Input: part model. Units: mm. Frame: model coordinates. A direction names the side the tool comes from. Round coordinates to 2 decimals unless told otherwise and drop trailing zeros. Loops run counter-clockwise (first coordinate to the right, second up) from the corner with the lowest first, then second, coordinate; pieces in that order, holes last. Notation, with made-up numbers: M -38,51.25 L 6,51.25 A20 cw 6,88.25 Z; hole C -2,73.5 d10. An arc over 180 degrees is marked long. Return JSON: item names as keys, results as strings. Group by question number.
1) Mould query, pull axis X, two halves, no side actions, for faces 1 (the face through (-24.31, -3.2, 15.17)), 2 (the face through (-14.635, 5.25, 17.269)), 3 (the face through (-5.546, -4.715, 34.699)), 4 (the face through (9.66, 19.845, 17.269)). Classes: +X half, -X half, draft (parallel to the pull), parting line (faces both ways), or undercut.
2) Section B-B (z = 23.5). Output: boundary loops of the cut face in (x, y), plus the area to 3 significant figures.
3) Access query for faces 5 (the face through (9.306, 1.042, 0.285)), 6 (the face through (12.705, -4.01, 3.715)), 7 (the face through (5, -1, 17)). Directions: +Z, -Z, +X, -X, +Y, -Y. A direction counts if a zero-diameter tool reaches every point of the face in a straight line with its end or side. Return the directions, or none.
4) Section A-A (z = 32). Output: boundary loops of the cut face in (x, y), plus the area to 3 significant figures.
5) Material intervals for line 1 (X direction, y = 2.5, z = 17.5); line 2 (X direction, y = 0, z = 31); line 3 (X direction, y = 6, z = 20), sorted ascending. Write a range as from..to.
6) Contact query for flat-ended pins moving along their axis: P1, Ø4, axis at y = 17.5, z = 12, coming from the -X side; P2, Ø3.5, axis at x = 5, z = 22.5, coming from the +Y side; P3, Ø2, axis at x = -10, z = 19.5, coming from the -Y side; P4, Ø6, axis at x = -11.5, y = 7, coming from the -Z side. Output: stop coordinate, or through.
from build123d import *

# Parameters (mm, degrees)
F0_W     = 7
F0_H     = 4
F1_DEPTH = 35
F5_DEPTH = 25
F2_W     = 37.6
F2_H     = 22
F6_DEPTH = 1.5
F7_R     = 1


with BuildPart() as f1:
    # F0 (on Top) → F1 (new body)
    with BuildSketch(Plane.XY):
        Polygon((-24.5947403937, 11), (-24.5947403937, -5), (13.0052596063, -5), (13.0052596063, 17.7735), (6.9012222925, 21.5526076059), (-5.5421815105, 0), align=None)
        Polygon((-20.5947403937, -1), (-20.5947403937, 4.0717967697), (-11.8101307029, -1), align=None, mode=Mode.SUBTRACT)
        with Locations((5.5052596063, 1)):
            Rectangle(F0_W, F0_H, mode=Mode.SUBTRACT)
    extrude(amount=F1_DEPTH)

    # F4 (on offset) → F5 (cut)
    with BuildSketch(Plane(origin=(0, 0, 5), x_dir=(1, 0, 0), z_dir=(0, 0, -1))):
        Polygon((13.0052596063, -22.1251103646), (13.0052596063, -3), (1.963371989, -3), align=None)
    extrude(amount=-F5_DEPTH, mode=Mode.SUBTRACT)

    # F2 (on face) → F6 (cut)
    with BuildSketch(Plane.XZ.offset(5)):
        with Locations((-5.7947403937, 15)):
            Rectangle(F2_W, F2_H)
    extrude(amount=-F6_DEPTH, mode=Mode.SUBTRACT)

    # F7
    f7_edges = [f1.edges().sort_by_distance(p)[0] for p in [
        (6.901222, 21.552608, 17.5),
        (-5.542182, 0, 17.5),
        (0.67952, 10.776304, 0),
        (0.67952, 10.776304, 35),
        (-24.59474, 11, 17.5),
        (-15.068461, 5.5, 0),
        (-15.068461, 5.5, 35),
        (-24.59474, 3, 0),
        (-5.79474, -5, 0),
        (13.00526, 6.38675, 0),
        (9.953241, 19.663054, 0),
        (-20.59474, 1.535898, 0),
        (-16.202436, 1.535898, 0),
        (-16.202436, -1, 0),
        (2.00526, 1, 0),
        (5.50526, 3, 0),
        (9.00526, 1, 0),
        (5.50526, -1, 0),
        (-24.59474, -5, 2),
        (-24.59474, -4.25, 4),
        (-24.59474, -3.5, 15),
        (-24.59474, -4.25, 26),
        (-24.59474, -5, 30.5),
        (-24.59474, 3, 35),
        (-5.79474, -5, 35),
        (13.00526, 6.38675, 35),
        (9.953241, 19.663054, 35),
        (-20.59474, 1.535898, 35),
        (-16.202436, 1.535898, 35),
        (-16.202436, -1, 35),
        (2.00526, 1, 35),
        (5.50526, 3, 35),
        (9.00526, 1, 35),
        (5.50526, -1, 35),
        (13.00526, 17.7735, 2.5),
        (13.00526, 10.38675, 5),
        (13.00526, 3, 17.5),
        (13.00526, 10.38675, 30),
        (13.00526, 17.7735, 32.5),
        (13.00526, -5, 30.5),
        (13.00526, -4.25, 26),
        (13.00526, -3.5, 15),
        (13.00526, -4.25, 4),
        (13.00526, -5, 2),
    ]]
    fillet(f7_edges, radius=F7_R)


solid = f1.part
Returned:
{
 "1": {"face 1": "-X half", "face 2": "undercut", "face 3": "draft", "face 4": "+X half"},
 "2": {"outline": "M -24.59,-2.5 A1 ccw -23.59,-3.5 L 12.01,-3.5 A1 ccw 13.01,-2.5 L 13.01,2 A1 ccw 12.01,3 L 9.01,3 L 9.01,-1 L 2.01,-1 L 2.01,3 L 1.96,3 L 11.15,18.92 L 7.78,21.01 A1 ccw 6.39,20.66 L -5.04,0.87 A1 cw -6.41,0.5 L -23.09,10.13 A1 ccw -24.59,9.27 Z; hole M -20.59,-1 L -11.81,-1 L -20.59,4.07 Z", "area": "337 mm^2"},
 "3": {"face 5": "-Z", "face 6": "+X, -Y", "face 7": "+Z, -Z"},
 "4": {"outline": "M -24.59,-4 A1 ccw -23.59,-5 L 12.01,-5 A1 ccw 13.01,-4 L 13.01,17.22 A1 ccw 12.53,18.07 L 7.78,21.01 A1 ccw 6.39,20.66 L -5.04,0.87 A1 cw -6.41,0.5 L -23.09,10.13 A1 ccw -24.59,9.27 Z; hole M -20.59,-1 L -11.81,-1 L -20.59,4.07 Z; hole M 2.01,-1 L 9.01,-1 L 9.01,3 L 2.01,3 Z", "area": "495 mm^2"},
 "5": {"line 1": "x = -24.59..-20.59, -17.87..-9.87, -4.1..2.01, 9.01..12.87", "line 2": "x = -24.59..-20.59, -13.54..2.01, 9.01..13.01", "line 3": "x = -24.59..-15.93, -2.08..3.7"},
 "6": {"P1": "stops at x = 3.41", "P2": "stops at y = 21.02", "P3": "stops at y = -3.5", "P4": "passes through"}
}
